For this review, take the finished solid that the model builds, in its own axes (mm). A direction names the side the tool comes from. Coordinates: 2 decimals unless noted, no trailing zeros. Write each loop counter-clockwise with the first axis right and the second up, starting at its lowest first coordinate (ties: lowest second). Pieces come first, ordered by that corner, then holes.
```python
from build123d import *

# Parameters (mm, degrees)
SKETCH1_W           = 122
SKETCH1_H           = 77
BOSS_EXTRUDE1_DEPTH = 9
SKETCH2_W           = 109
SKETCH2_H           = 66
CUT_EXTRUDE1_DEPTH  = 1
BOSS_EXTRUDE2_DEPTH = 2
SKETCH4_R           = 1.75
CUT_EXTRUDE3_DEPTH  = 4
SKETCH5_W           = 12
SKETCH5_H           = 4
SKETCH5_W_2         = 20
SKETCH5_H_2         = 5
CUT_EXTRUDE4_DEPTH  = 2


with BuildPart() as part:
    # Sketch1 → Boss-Extrude1 (new body)
    with BuildSketch(Plane(origin=(0, 0, 0), x_dir=(1, 0, 0), z_dir=(0, 1, 0))):
        with Locations((61, 38.5)):
            Rectangle(SKETCH1_W, SKETCH1_H)
    extrude(amount=BOSS_EXTRUDE1_DEPTH)

    # Sketch2 → Cut-Extrude1 (cut)
    with BuildSketch(Plane(origin=(0, 9, 0), x_dir=(1, 0, 0), z_dir=(0, 1, 0))):
        with Locations((61, 38.5)):
            Rectangle(SKETCH2_W, SKETCH2_H)
    extrude(amount=-CUT_EXTRUDE1_DEPTH, mode=Mode.SUBTRACT)

    # Sketch3 → Boss-Extrude2 (add)
    with BuildSketch(Plane.XZ):
        with BuildLine():
            Line((0, -81.66), (0, -72.34))
            ThreePointArc((0, -72.34), (4, -68.34), (8, -72.34))
            Line((8, -72.34), (8, -81.66))
            ThreePointArc((8, -81.66), (4, -85.66), (0, -81.66))
        make_face()
        with BuildLine():
            Line((122, -81.66), (122, -72.34))
            ThreePointArc((122, -72.34), (118, -68.34), (114, -72.34))
            Line((114, -72.34), (114, -81.66))
            ThreePointArc((114, -81.66), (118, -85.66), (122, -81.66))
        make_face()
        with BuildLine():
            Line((0, 4.66), (0, -4.66))
            ThreePointArc((0, -4.66), (4, -8.66), (8, -4.66))
            Line((8, -4.66), (8, 4.66))
            ThreePointArc((8, 4.66), (4, 8.66), (0, 4.66))
        make_face()
        with BuildLine():
            Line((122, 4.66), (122, -4.66))
            ThreePointArc((122, -4.66), (118, -8.66), (114, -4.66))
            Line((114, -4.66), (114, 4.66))
            ThreePointArc((114, 4.66), (118, 8.66), (122, 4.66))
        make_face()
    extrude(amount=-BOSS_EXTRUDE2_DEPTH)

    # Sketch4 → Cut-Extrude3 (cut)
    with BuildSketch(Plane.XZ):
        with Locations(Location((4, -81.66, 0), (0, 0, 270))):
            Circle(SKETCH4_R)
        with Locations(Location((118, -81.66, 0), (0, 0, 90))):
            Circle(SKETCH4_R)
        with Locations(Location((4, 4.66, 0), (0, 0, 90))):
            Circle(SKETCH4_R)
        with Locations(Location((118, 4.66, 0), (0, 0, 270))):
            Circle(SKETCH4_R)
    extrude(amount=-CUT_EXTRUDE3_DEPTH, mode=Mode.SUBTRACT)

    # Sketch5 → Cut-Extrude4 (cut)
    with BuildSketch(Plane(origin=(122, 0, 0), x_dir=(0, 0, -1), z_dir=(1, 0, 0))):
        with Locations((67, 5)):
            Rectangle(SKETCH5_W, SKETCH5_H)
        with Locations((47, 4.5)):
            Rectangle(SKETCH5_W_2, SKETCH5_H_2)
    extrude(amount=-CUT_EXTRUDE4_DEPTH, mode=Mode.SUBTRACT)


solid = part.part
```
1) For L1, parallel to X at y = 1.25, z = -81.66; L2, parallel to Z at x = 118, y = 1.35; L3, parallel to X at y = 8.25, z = -32.5, list the stretches that pass through material, from the lowest coordinate up.
2) The part is to be moulded in two halves that separate along X. For faces 1 (the face through (4.08, 0.99, -79.91)), 2 (the face through (120, 5, -47)), 3 (the face through (47, 9, -4)), say which applies: pulls with the +X half, pulls with the -X half, needs draft (parallel to the pull), parting line crosses it, or undercut.
3) Consider section D-D (x = 71.5). Give the boundary of the cut face in (y, z).
4) Consider section A-A (x = 4). Give the boundary of the cut face in (y, z).
5) Consider section C-C (z = -42.5). Give the boundary of the cut face in (x, y).
6) Consider section B-B (y = 4.5). Give the boundary of the cut face in (x, z).
7) Clearance check with flat-ended pins moving along their axes: P1, Ø4, axis at x = 76, z = -50, coming from the +Y side; P2, Ø3, axis at x = 65.5, y = 1, coming from the +Z side; P3, Ø4, axis at x = 119.5, z = 5, coming from the +Y side. State where each tip first meets the part, or that it passes through.
8) Tool access review of faces 4 (the face through (60, 8, -39)), 5 (the face through (4, 2, -79)), 6 (the face through (4, 2, 2)): name each direction out of +Z, -Z, +X, -X, +Y, -Y from which nothing blocks a thin tool from reaching the whole face with its end or side.
Results:
1. L1: x = 0 to 2.25, 5.75 to 8, 114 to 116.25, 119.75 to 122
1. L2: z = -85.66 to -83.41, -79.91 to 2.91, 6.41 to 8.66
1. L3: x = 0 to 6.5, 115.5 to 122
2. face 1: undercut
2. face 2: pulls with the +X half
2. face 3: needs draft
3. outline: (0, -77) - (9, -77) - (9, -71.5) - (8, -71.5) - (8, -5.5) - (9, -5.5) - (9, 0) - (0, 0) - close
4. outline: (0, -85.66) - (2, -85.66) - (2, -83.41) - (0, -83.41) - close; (0, -79.91) - (2, -79.91) - (2, -77) - (9, -77) - (9, 0) - (2, 0) - (2, 2.91) - (0, 2.91) - close; (0, 6.41) - (2, 6.41) - (2, 8.66) - (0, 8.66) - close
5. outline: (0, 0) - (122, 0) - (122, 2) - (120, 2) - (120, 7) - (122, 7) - (122, 9) - (115.5, 9) - (115.5, 8) - (6.5, 8) - (6.5, 9) - (0, 9) - close
6. outline: (0, -77) - (122, -77) - (122, -73) - (120, -73) - (120, -61) - (122, -61) - (122, -57) - (120, -57) - (120, -37) - (122, -37) - (122, 0) - (0, 0) - close
7. P1: stops at y = 8
7. P2: stops at z = 0
7. P3: stops at y = 2
8. face 4: +Y
8. face 5: -Z, +X, -X, +Y
8. face 6: +Z, +X, -X, +Y
